The listing builds one solid part. Answer for the finished solid, in the listing's coordinates (mm). Face numbers are marked on the shaded views. A direction names the side the tool comes from. Give positions to 0.01 mm unless a question says otherwise; leave off trailing zeros. Write each loop counter-clockwise with the first axis right and the second up, starting at its lowest first coordinate (ties: lowest second). Pieces come first, ordered by that corner, then holes. Notation, with made-up numbers: (82.25, -26) - (107.25, -26) arc R22 cw to (107.25, -13) - close; hole circle Ø10 at (24, 26.25). An arc over 180 degrees is marked (long way). One line per item, written item: value. Start each with the question number.
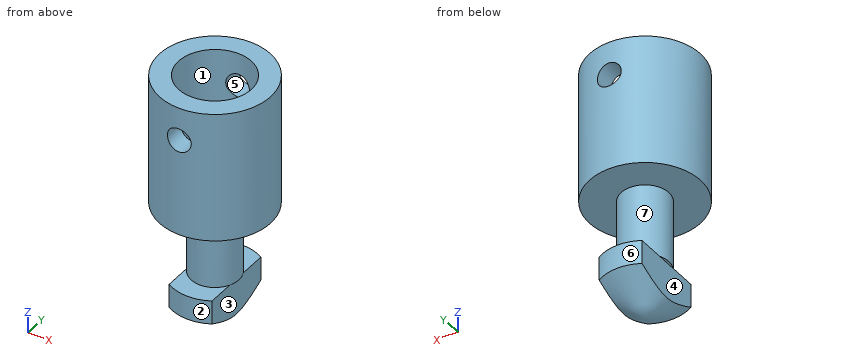
from build123d import *

# Parameters (mm, degrees)
CUT_EXTRUDE1_START      = -8.5
SKETCH2_W               = 5
SKETCH2_H               = 10
CUT_EXTRUDE1_DEPTH      = 3.542335768
CUT_EXTRUDE2_DEPTH      = 12.042335768
CUT_EXTRUDE2_DEPTH_BACK = 12.042335768
SKETCH3_R               = 0.5


with BuildPart() as part:
    # Sketch1 → Revolve1 (revolve)
    with BuildSketch(Plane(origin=(0, 0, 0), x_dir=(0, 0, -1), z_dir=(1, 0, 0)), mode=Mode.PRIVATE) as revolve1_sk:
        Polygon((0, 2.33), (5.5, 2.33), (5.5, 1), (8.5, 1), (8.5, 1.8), (9.5, 1.8), (10.539230485, 0), (4, 0), (4, 1.53), (0, 1.53), align=None)
    revolve(revolve1_sk.sketch.rotate(Axis((0, 0, 2.965537871), (0, 0, -1)), 180), axis=Axis((0, 0, 2.965537871), (0, 0, -1)))

    # Sketch2 → Cut-Extrude1 (cut, through all)
    with BuildSketch(Plane.XY.offset(CUT_EXTRUDE1_START)):
        with Locations((3.4, 0)):
            Rectangle(SKETCH2_W, SKETCH2_H)
        with Locations((-3.4, 0)):
            Rectangle(SKETCH2_W, SKETCH2_H)
    extrude(amount=-CUT_EXTRUDE1_DEPTH, mode=Mode.SUBTRACT)

    # Sketch3 → Cut-Extrude2 (cut, two sides: drawn at the far end of the back side and taken through both)
    with BuildSketch(Plane(origin=(0, 0, 0), x_dir=(1, 0, 0), z_dir=(0, 1, 0)).offset(-CUT_EXTRUDE2_DEPTH_BACK)):
        with Locations(Location((0, 1.4, 0), (0, 0, 270))):
            Circle(SKETCH3_R)
    extrude(amount=CUT_EXTRUDE2_DEPTH + CUT_EXTRUDE2_DEPTH_BACK, mode=Mode.SUBTRACT)


solid = part.part
Item 1: Find section C-C on x = -1.3. Determine the outline of the cut face in (y, z), plus the area to 3 significant figures.
Item 2: For the marked faces 4, 5, 6 and 7, determine the directions among +Z, -Z, +X, -X, +Y, -Y from which every point of the face is accessible in a straight line to the end or side of a thin tool.
Item 3: Find section A-A on z = -1.4. Determine the outline of the cut face in (x, y).
Item 4: The mould has two halves that part along X. Classify the marked faces 1, 2 and 3: +X half, -X half, draft (parallel to the pull), parting line (faces both ways), or undercut.
Item 5: Each of these flat-tipped pins is pushed along its axis until it touches: pin 1 Ø1.2 at (y, z) = (1, -9) entering from +X; pin 2 Ø0.8 at (y, z) = (-0.5, -9) entering from -X; pin 3 Ø1.5 at (x, z) = (-1, -2) entering from -Y. Where does it stop, or does it pass through?
Item 6: Find section D-D on y = 1.7. Give the number of separate pieces and of enclosed holes in the cut face, plus the area to 3 significant figures.
Item 7: Straight lines are drawn through the part: line 1 along X through (y, z) = (0, -1.9); line 2 along Z through (x, y) = (0, 1.9); line 3 along Y through (x, z) = (0.2, -3.25). For each, find the intervals that lie inside material, in ascending order.
Item 8: Find section B-B on z = -3.25. Determine the outline of the cut face in (x, y), plus the area to 3 significant figures.
Values:
1. outline: (-1.93, -5.5) - (1.93, -5.5) - (1.93, 0) - (0.81, 0) - (0.81, -4) - (-0.81, -4) - (-0.81, 0) - (-1.93, 0) - close
1. area: 14.8 mm^2
2. face 4: -Z, -X, +Y, -Y
2. face 5: +Y, -Y
2. face 6: -Z, +Y
2. face 7: none
3. outline: (-0.5, -2.28) - (-0.5, -1.45) arc R1.53 cw to (-0.5, 1.45) - (-0.5, 2.28) arc R2.33 ccw to start; (0.5, -2.28) arc R2.33 ccw to (0.5, 2.28) - (0.5, 1.45) arc R1.53 cw to (0.5, -1.45) - close
4. face 1: undercut
4. face 2: parting line
4. face 3: +X half
5. pin 1: x = 0.9
5. pin 2: x = -0.9
5. pin 3: y = -2.32
6. separate pieces: 2
6. enclosed holes: 1
6. area: 18.0 mm^2
7. line 1: -2.33 to -1.53, 1.53 to 2.33
7. line 2: -5.5 to -1.9, -0.9 to 0
7. line 3: -2.32 to -1.52, 1.52 to 2.32
8. outline: circle Ø4.66 at (0, 0); hole circle Ø3.06 at (0, 0)
8. area: 9.70 mm^2
